from build123d import *

# Parameters (mm, degrees)
BOSS_EXTRUDE1_DEPTH     = 25.5
SKETCH2_R               = 4.5
CUT_EXTRUDE1_DEPTH      = 25
SKETCH3_R               = 1.5
CUT_EXTRUDE2_DEPTH      = 10
SKETCH4_R               = 5
CUT_EXTRUDE3_DEPTH      = 2
CUT_EXTRUDE4_DEPTH      = 3
CUT_EXTRUDE5_DEPTH      = 3
SKETCH7_R               = 4.5
CUT_EXTRUDE6_DEPTH      = 2
CUT_EXTRUDE7_DEPTH      = 108.685885798
CUT_EXTRUDE7_DEPTH_BACK = 108.685885798
SKETCH8_R               = 1.5
SKETCH9_R               = 5
CUT_EXTRUDE8_DEPTH      = 10
BOSS_EXTRUDE2_DEPTH     = 25.5


with BuildPart() as part:
    # Sketch1 → Boss-Extrude1 (new body)
    with BuildSketch(Plane(origin=(0, 0, 0), x_dir=(1, 0, 0), z_dir=(0, 1, 0))):
        Polygon((6, -6), (55, -6), (55, -85), (61, -85), (61, 60), (55, 60), (55, 0), (6, 0), (6, 60), (0, 60), (0, -85), (6, -85), align=None)
    extrude(amount=BOSS_EXTRUDE1_DEPTH)

    # Sketch2 → Cut-Extrude1 (cut)
    with BuildSketch(Plane(origin=(6, 0, 0), x_dir=(0, 0, -1), z_dir=(1, 0, 0))):
        with Locations((-71, 12.75)):
            Circle(SKETCH2_R)
    extrude(amount=-CUT_EXTRUDE1_DEPTH, mode=Mode.SUBTRACT)

    # Sketch3 → Cut-Extrude2 (cut)
    with BuildSketch(Plane.ZY.offset(-55)):
        with Locations((71, 12.75)):
            Circle(SKETCH3_R)
    extrude(amount=-CUT_EXTRUDE2_DEPTH, mode=Mode.SUBTRACT)

    # Sketch4 → Cut-Extrude3 (cut)
    with BuildSketch(Plane(origin=(61, 0, 0), x_dir=(0, 0, -1), z_dir=(1, 0, 0))):
        with Locations((-71, 12.75)):
            Circle(SKETCH4_R)
    extrude(amount=-CUT_EXTRUDE3_DEPTH, mode=Mode.SUBTRACT)

    # Sketch5 → Cut-Extrude4 (cut)
    with BuildSketch(Plane.ZY.offset(-55)):
        with BuildLine():
            Line((71, 19.25), (54, 15.75))
            ThreePointArc((54, 15.75), (51, 12.75), (54, 9.75))
            Line((54, 9.75), (71, 6.25))
            ThreePointArc((71, 6.25), (77.5, 12.75), (71, 19.25))
        make_face()
    extrude(amount=-CUT_EXTRUDE4_DEPTH, mode=Mode.SUBTRACT)

    # Sketch6 → Cut-Extrude5 (cut)
    with BuildSketch(Plane.ZY.offset(-55)):
        with BuildLine():
            Line((-29, 9.75), (-46, 6.25))
            ThreePointArc((-46, 6.25), (-52.5, 12.75), (-46, 19.25))
            Line((-46, 19.25), (-29, 15.75))
            ThreePointArc((-29, 15.75), (-26, 12.75), (-29, 9.75))
        make_face()
    extrude(amount=-CUT_EXTRUDE5_DEPTH, mode=Mode.SUBTRACT)

    # Sketch7 → Cut-Extrude6 (cut)
    with BuildSketch(Plane(origin=(61, 0, 0), x_dir=(0, 0, -1), z_dir=(1, 0, 0))):
        with Locations((46, 12.75)):
            Circle(SKETCH7_R)
    extrude(amount=-CUT_EXTRUDE6_DEPTH, mode=Mode.SUBTRACT)

    # Sketch8 → Cut-Extrude7 (cut, two sides: drawn at the far end of the back side and taken through both)
    with BuildSketch(Plane(origin=(61, 0, 0), x_dir=(0, 0, -1), z_dir=(1, 0, 0)).offset(-CUT_EXTRUDE7_DEPTH_BACK)):
        with Locations((46, 12.75)):
            Circle(SKETCH8_R)
    extrude(amount=CUT_EXTRUDE7_DEPTH + CUT_EXTRUDE7_DEPTH_BACK, mode=Mode.SUBTRACT)

    # Sketch9 → Cut-Extrude8 (cut)
    with BuildSketch(Plane.ZY):
        with Locations((-46, 12.75)):
            Circle(SKETCH9_R)
    extrude(amount=-CUT_EXTRUDE8_DEPTH, mode=Mode.SUBTRACT)

    # Sketch10 → Boss-Extrude2 (add)
    with BuildSketch(Plane(origin=(0, 25.5, 0), x_dir=(1, 0, 0), z_dir=(0, 1, 0))):
        Polygon((9, -6), (6, -6), (6, -9), align=None)
        Polygon((6, 0), (6, 3), (9, 0), align=None)
        Polygon((52, 0), (55, 0), (55, 3), align=None)
        Polygon((55, -6), (55, -9), (52, -6), align=None)
    extrude(amount=-BOSS_EXTRUDE2_DEPTH)


solid = part.part
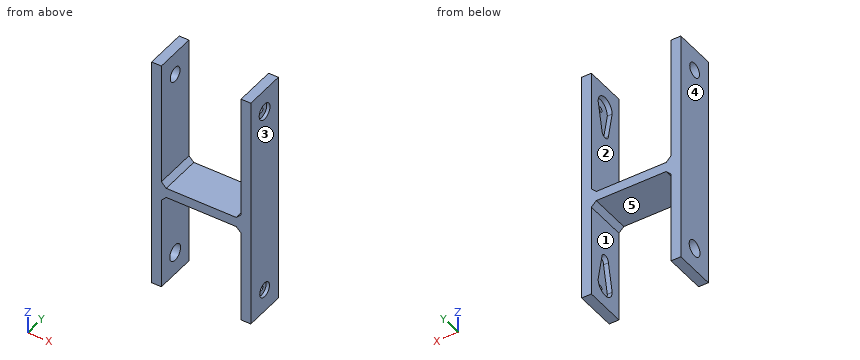
Design review of the part built by this model. Coordinates are the model's own, in mm. Face numbers are marked on the shaded views. A direction names the side the tool comes from. Round coordinates to 2 decimals unless told otherwise and drop trailing zeros. Write each loop counter-clockwise with the first axis right and the second up, starting at its lowest first coordinate (ties: lowest second). Pieces come first, ordered by that corner, then holes.
Item 1: Consider section C-C on y = 2.75. Give the boundary of the cut face in (x, z).
Item 2: Wall thickness on L1, parallel to X at y = 17, z = -53.5; L2, parallel to X at y = 9.5, z = 62; L3, parallel to Y at x = 58.45, z = -46: over which ranges is each line inside the solid? List them lowest first.
Item 3: Draft analysis for pull direction X (two halves, no side actions). For the marked faces 3, 4 and 5, state which applies: released by +X, released by -X, zero draft, split by the parting line, or undercut.
Item 4: Consider section D-D on x = 24. Give the boundary of the cut face in (y, z), and give its area (3 significant figures).
Item 5: For the marked faces 1 and 2, list the 3-axis set-ups (+Z, -Z, +X, -X, +Y, -Y) from which the entire face can be reached by the end or side of a thin tool; tool diameter is ignored.
Item 6: Consider section B-B on y = 12.75. Count the separate pieces of the cut face and the enclosed holes in it, and give its area (4 significant figures).
Item 7: Consider section A-A on z = -1.5. Give the boundary of the cut face in (x, y).
Item 8: For pin 1 Ø13 at (x, y) = (35, 6.5) entering from +Z; pin 2 Ø12 at (y, z) = (9.5, 33) entering from -X; pin 3 Ø1.8 at (y, z) = (12.75, 71) entering from -X; pin 4 Ø3 at (x, y) = (53, 5.5) entering from -Z, all flat-tipped, find the tip position at first contact; note any pin that passes through.
Check values:
1. outline: (0, -60) - (6, -60) - (6, -3) - (9, 0) - (52, 0) - (55, -3) - (55, -60) - (61, -60) - (61, 85) - (55, 85) - (55, 9) - (52, 6) - (9, 6) - (6, 9) - (6, 85) - (0, 85) - close
2. L1: x = 0 to 6, 55 to 61
2. L2: x = 0 to 6, 58 to 61
2. L3: y = 0 to 11.25, 14.25 to 25.5
3. face 3: released by +X
3. face 4: released by -X
3. face 5: undercut
4. outline: (0, 0) - (25.5, 0) - (25.5, 6) - (0, 6) - close
4. area: 153 mm2
5. face 1: -Z, +Y, -Y
5. face 2: +Z, +Y, -Y
6. separate pieces: 5
6. enclosed holes: 0
6. area: 1,735 mm2
7. outline: (0, 0) - (7.5, 0) - (7.5, 25.5) - (0, 25.5) - close; (53.5, 0) - (61, 0) - (61, 25.5) - (53.5, 25.5) - close
8. pin 1: stops at z = 6
8. pin 2: stops at x = 0
8. pin 3: passes through
8. pin 4: stops at z = -2.5
